```python
from build123d import *

# Parameters (mm, degrees)
BOSS_EXTRUDE1_DEPTH = 2.3
FILLET1_R           = 3
BOSS_EXTRUDE2_DEPTH = 2
FILLET2_R           = 0.5


with BuildPart() as part:
    # Sketch2 → Boss-Extrude1 (new body)
    with BuildSketch(Plane.XY):
        with BuildLine():
            ThreePointArc((-11.15, 0), (-8.220642305, 7.532830815), (-0.971786532, 11.107570884))
            Line((-0.971786532, 11.107570884), (-1.122130188, 12.826006738))
            ThreePointArc((-1.122130188, 12.826006738), (-9.492445711, 8.698223923), (-12.875, 0))
            Line((-12.875, 0), (-11.15, 0))
        make_face()
        with BuildLine():
            ThreePointArc((-10, 0), (-7.372773368, 6.755902076), (-0.871557427, 9.961946981))
            Line((-0.871557427, 9.961946981), (-0.971786532, 11.107570884))
            ThreePointArc((-0.971786532, 11.107570884), (-8.220642305, 7.532830815), (-11.15, 0))
            Line((-11.15, 0), (-10, 0))
        make_face()
        with BuildLine():
            Line((-0.971786532, 11.107570884), (-0.871557427, 9.961946981))
            ThreePointArc((-0.871557427, 9.961946981), (6.755902076, 7.372773368), (10, 0))
            Line((10, 0), (11.15, 0))
            ThreePointArc((11.15, 0), (10.885700479, 2.413301695), (10.105331825, 4.712193618))
            ThreePointArc((10.105331825, 4.712193618), (5.575, 9.656183252), (-0.971786532, 11.107570884))
        make_face()
        with BuildLine():
            ThreePointArc((10, 0), (7.372773368, -6.755902076), (0.871557427, -9.961946981))
            Line((0.871557427, -9.961946981), (0.971786532, -11.107570884))
            ThreePointArc((0.971786532, -11.107570884), (8.220642305, -7.532830815), (11.15, 0))
            Line((11.15, 0), (10, 0))
        make_face()
        with BuildLine():
            Line((0.971786532, -11.107570884), (0.871557427, -9.961946981))
            ThreePointArc((0.871557427, -9.961946981), (-6.755902076, -7.372773368), (-10, 0))
            Line((-10, 0), (-11.15, 0))
            ThreePointArc((-11.15, 0), (-7.532830815, -8.220642305), (0.971786532, -11.107570884))
        make_face()
        with BuildLine():
            ThreePointArc((11.15, 0), (8.220642305, -7.532830815), (0.971786532, -11.107570884))
            Line((0.971786532, -11.107570884), (1.122130188, -12.826006738))
            ThreePointArc((1.122130188, -12.826006738), (9.492445711, -8.698223923), (12.875, 0))
            Line((12.875, 0), (11.15, 0))
        make_face()
    extrude(amount=BOSS_EXTRUDE1_DEPTH)

    # Fillet1
    # the kernel refuses this fillet: 3 mm, written as the material it takes off along each edge
    with BuildSketch(Plane(origin=(-1.757754934, 20.091230835, 2.3), x_dir=(0, 0, -1), z_dir=(0.08715574274757223, -0.9961946980917531, 0))) as fillet1_piece_1_section:
        with BuildLine():
            CenterArc((3, -2.917190429), FILLET1_R, 103.493398822, 76.506601178)
            Line((0, -2.917190429), (0, 0))
            Line((0, 0), (2.3, 0))
        make_face()
    fillet1_piece_1 = extrude(amount=16.310952146, mode=Mode.PRIVATE)
    fillet1_piece_1 = fillet1_piece_1 - Plane(origin=(0, 0, 1.660555485), x_dir=(1, 0, 0), z_dir=(0, 0, -1)) * Cylinder(11.15, 45, mode=Mode.PRIVATE)
    add(fillet1_piece_1, mode=Mode.SUBTRACT)
    with BuildSketch(Plane(origin=(0.336161785, -3.842346787, 2.3), x_dir=(0.9961946980917454, 0.08715574274765826, 0), z_dir=(0.08715574274765828, -0.9961946980917455, 0))) as fillet1_piece_2_section:
        with BuildLine():
            CenterArc((2.917190429, -3), FILLET1_R, 90, 76.506601178)
            Line((0, -2.3), (0, 0))
            Line((0, 0), (2.917190429, 0))
        make_face()
    fillet1_piece_2 = extrude(amount=16.310952146, mode=Mode.PRIVATE)
    fillet1_piece_2 = fillet1_piece_2 - Plane(origin=(0, 0, 1.660555485), x_dir=(1, 0, 0), z_dir=(0, 0, -1)) * Cylinder(11.15, 45, mode=Mode.PRIVATE)
    add(fillet1_piece_2, mode=Mode.SUBTRACT)

    # Sketch3 → Boss-Extrude2 (add)
    with BuildSketch(Plane.XY.offset(2.3)):
        with BuildLine():
            ThreePointArc((-10, 0), (-9.84807753, 1.736481777), (-9.396926208, 3.420201433))
            Line((-9.396926208, 3.420201433), (-12.098542493, 4.403509345))
            ThreePointArc((-12.098542493, 4.403509345), (-12.67939982, 2.235720287), (-12.875, 0))
            Line((-12.875, 0), (-11.15, 0))
            Line((-11.15, 0), (-10, 0))
        make_face()
        with BuildLine():
            ThreePointArc((10, 0), (9.84807753, -1.736481777), (9.396926208, -3.420201433))
            Line((9.396926208, -3.420201433), (12.098542493, -4.403509345))
            ThreePointArc((12.098542493, -4.403509345), (12.67939982, -2.235720287), (12.875, 0))
            Line((12.875, 0), (11.15, 0))
            Line((11.15, 0), (10, 0))
        make_face()
    extrude(amount=BOSS_EXTRUDE2_DEPTH)

    # Fillet2
    fillet2_edges = [part.edges().sort_by_distance(p)[0] for p in [
        (-11.4375, 0, 4.3),
        (-9.84807753, 1.736481777, 4.3),
        (-10.74773435, 3.911855389, 4.3),
        (-12.67939982, 2.235720287, 4.3),
        (11.4375, 0, 4.3),
        (9.84807753, -1.736481777, 4.3),
        (10.74773435, -3.911855389, 4.3),
        (12.67939982, -2.235720287, 4.3),
    ]]
    fillet(fillet2_edges, radius=FILLET2_R)


solid = part.part
```
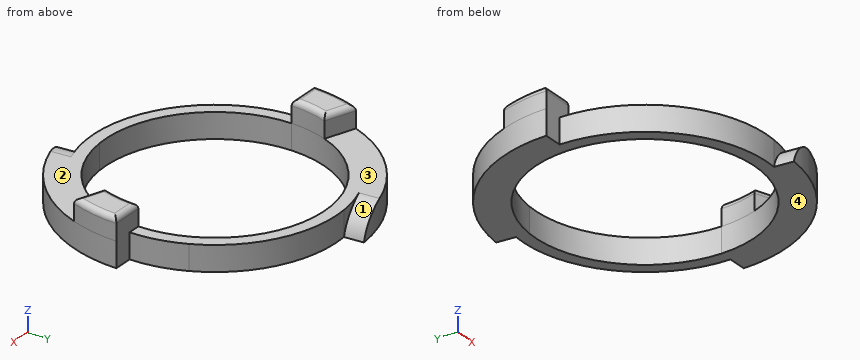
Geometry check sheet. Reference: the model listing, model coordinates, mm. Face numbers are marked on the shaded views. A direction names the side the tool comes from. Coordinates: 2 decimals unless noted, no trailing zeros. Order: outer loops, then holes, each group sorted by start corner. A loop starts at its lowest first (then second) coordinate and runs counter-clockwise, first axis right, second up. Notation, with made-up numbers: (79.25, -1.75) - (125.25, -1.75) arc R25 cw to (125.25, 28.25) - close; hole circle Ø7 at (89, 20). An arc over 180 degrees is marked (long way). Answer in a Markdown table with one row per item. Add a question column.
1. Access from +Z, -Z, +X, -X, +Y, -Y to the whole of each face (thin tool, end or side, straight path). Record for the marked faces 1, 2, 3 and 4.
2. Gauge pin test, flat ends, axial feed: pin 1 Ø5 at (x, y) = (-4, -10) entering from +Z; pin 2 Ø0.9 at (x, z) = (-12, 1.5) entering from -Y. Record the tip position at first contact, or that the pin passes through.
3. Material ranges on L1, parallel to Z at x = -6.25, y = 9; L2, parallel to Y at x = -9.25, z = 1.3; L3, parallel to Y at x = 4, z = 1.2, recorded low to high. Write a range as [from, to].
4. Section check B-B (x = 7.75). Enter the section's corners in (y, z).
5. Section check C-C (z = 1.7). Enter the section's corners in (x, y) (3 decimals).
6. Section check A-A (y = 9). Enter the section's corners in (x, z), plus the area to 3 significant figures.
Data:
| question | item | result |
|---|---|---|
| 1 | face 1 | +Z, +Y |
| 1 | face 2 | +Z, -X, -Y |
| 1 | face 3 | +Z, +X, +Y |
| 1 | face 4 | -Z, +X, -X, +Y, -Y |
| 2 | pin 1 | stops at z = 2.3 |
| 2 | pin 2 | stops at y = 0 |
| 3 | L1 | z = [0, 2.3] |
| 3 | L2 | y = [-6.23, -3.8], [3.8, 8.96] |
| 3 | L3 | y = [-12.24, -9.17], [9.17, 10.41] |
| 4 | outline | (-10.28, 0) - (-6.32, 0) - (-6.32, 2.3) - (-10.28, 2.3) - close; (6.32, 0) - (8.02, 0) - (8.02, 2.3) - (6.32, 2.3) - close |
| 5 | outline | (-12.875, 0) - (-11.15, 0) arc R11.15 ccw to (2.08, -10.954) - (2.231, -12.68) arc R12.875 ccw to (12.875, 0) - (11.15, 0) arc R11.15 ccw to (-2.08, 10.954) - (-2.231, 12.68) arc R12.875 ccw to start; hole circle Ø20 at (0, 0) |
| 6 | outline | (-9.21, 0) - (-4.36, 0) - (-4.36, 2.3) - (-9.21, 2.3) - close; (4.36, 0) - (6.58, 0) - (6.58, 2.3) - (4.36, 2.3) - close |
| 6 | area | 16.3 mm² |
